from build123d import *

# Parameters (mm, degrees)
BOSS_EXTRUDE1_DEPTH = 3
SKETCH2_R           = 1.6
CUT_EXTRUDE1_DEPTH  = 7
CHAMFER1_SIZE       = 3.5
FILLET1_R           = 0.5


with BuildPart() as part:
    # Sketch1 → Boss-Extrude1 (new body, symmetric)
    with BuildSketch(Plane.XY):
        Polygon((-7, 0), (7, 0), (7, -18.5), (12, -18.5), (6.803847577, -27.5), (-6.803847577, -27.5), (-12, -18.5), (-7, -18.5), align=None)
    extrude(amount=BOSS_EXTRUDE1_DEPTH, both=True)

    # Sketch2 → Cut-Extrude1 (cut, through all)
    with BuildSketch(Plane.XY.offset(3)):
        with Locations((0, -6.3)):
            Circle(SKETCH2_R)
    extrude(amount=-CUT_EXTRUDE1_DEPTH, mode=Mode.SUBTRACT)

    # Chamfer1
    chamfer1_edges = [part.edges().sort_by_distance(p)[0] for p in [
        (-7, 0, 0),
        (7, 0, 0),
    ]]
    chamfer(chamfer1_edges, length=CHAMFER1_SIZE)

    # Fillet1
    fillet1_edges = [part.edges().sort_by_distance(p)[0] for p in [
        (12, -18.5, 0),
        (6.803847577, -27.5, 0),
        (-6.803847577, -27.5, 0),
        (-12, -18.5, 0),
    ]]
    fillet(fillet1_edges, radius=FILLET1_R)


solid = part.part
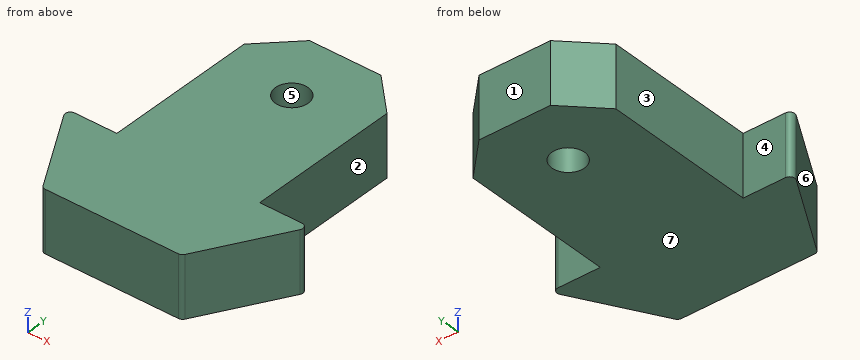
For this review, take the finished solid that the model builds, in its own axes (mm). Face numbers are marked on the shaded views. A direction names the side the tool comes from. Coordinates: 2 decimals unless noted, no trailing zeros. Loops run counter-clockwise (first coordinate to the right, second up) from the corner with the lowest first, then second, coordinate; pieces in that order, holes last. Notation, with made-up numbers: (8.5, 48) - (42.5, 48) arc R11 ccw to (42.5, 58) - close; hole circle Ø1 at (17.25, 86). An arc over 180 degrees is marked (long way). Use a Markdown table: item, result. Add a question column.
Item 1: We need section C-C (y = -6.3). Give the boundary of the cut face in (x, z).
Item 2: Insertion check: pin 1 Ø1.8 at (y, z) = (-12, -1) entering from -X; pin 2 Ø3.5 at (x, z) = (8, 0) entering from +Y; pin 3 Ø1.8 at (y, z) = (-10, 0) entering from +X. Each pin has a flat end and moves straight along its axis. Give the tip position at first contact, or say it passes through.
Item 3: We need section A-A (x = 0). Give the boundary of the cut face in (y, z), and give its area (3 significant figures).
Item 4: We need section B-B (z = 1.85). Give the boundary of the cut face in (x, y).
Item 5: Tool access review of the marked faces 1, 2 and 3: name each direction out of +Z, -Z, +X, -X, +Y, -Y from which nothing blocks a thin tool from reaching the whole face with its end or side.
Item 6: For line 1 (Y direction, x = 0, z = -0.9); line 2 (X direction, y = -5.5, z = -1.65); line 3 (Y direction, x = -1, z = 0), list the stretches that pass through material, from the lowest coordinate up.
Item 7: Mouldability with a two-part tool opening along Y and no side actions: class the marked faces 4, 5, 6 and 7 as pulls with the +Y half, pulls with the -Y half, needs draft (parallel to the pull), parting line crosses it, or undercut.
Item 8: We need section D-D (y = -2.5). Give the boundary of the cut face in (x, z).
Results list:
| question | item | result |
|---|---|---|
| 1 | outline | (-7, -3) - (-1.6, -3) - (-1.6, 3) - (-7, 3) - close; (1.6, -3) - (7, -3) - (7, 3) - (1.6, 3) - close |
| 2 | pin 1 | stops at x = -7 |
| 2 | pin 2 | stops at y = -2.75 |
| 2 | pin 3 | stops at x = 7 |
| 3 | outline | (-27.5, -3) - (-7.9, -3) - (-7.9, 3) - (-27.5, 3) - close; (-4.7, -3) - (0, -3) - (0, 3) - (-4.7, 3) - close |
| 3 | area | 146 mm^2 |
| 4 | outline | (-11.57, -19.25) - (-6.95, -27.25) arc R0.5 ccw to (-6.52, -27.5) - (6.52, -27.5) arc R0.5 ccw to (6.95, -27.25) - (11.57, -19.25) arc R0.5 ccw to (11.13, -18.5) - (7, -18.5) - (7, -3.5) - (3.5, 0) - (-3.5, 0) - (-7, -3.5) - (-7, -18.5) - (-11.13, -18.5) arc R0.5 ccw to start; hole circle Ø3.2 at (0, -6.3) |
| 5 | face 1 | +Z, -Z, +X, -X, +Y |
| 5 | face 2 | +Z, -Z, +X, +Y |
| 5 | face 3 | +Z, -Z, -X, +Y |
| 6 | line 1 | y = -27.5 to -7.9, -4.7 to 0 |
| 6 | line 2 | x = -7 to -1.39, 1.39 to 7 |
| 6 | line 3 | y = -27.5 to -7.55, -5.05 to 0 |
| 7 | face 4 | pulls with the +Y half |
| 7 | face 5 | undercut |
| 7 | face 6 | pulls with the -Y half |
| 7 | face 7 | needs draft |
| 8 | outline | (-6, -3) - (6, -3) - (6, 3) - (-6, 3) - close |
